```python
from build123d import *

# Parameters (mm, degrees)
SKETCH1_R           = 6.8961
SKETCH1_R_2         = 2.3241
BOSS_EXTRUDE1_DEPTH = 2.794
SKETCH2_R           = 2.3241
BOSS_EXTRUDE2_DEPTH = 0.762
BOSS_EXTRUDE3_DEPTH = 1.651
SKETCH5_R           = 8.206879239
SKETCH5_R_2         = 3.9875
CUT_EXTRUDE1_DEPTH  = 11.144891642
SKETCH6_R           = 4.9875
SKETCH6_R_2         = 3.9875
BOSS_EXTRUDE4_DEPTH = 1
FILLET1_R           = 0.2
SKETCH7_R           = 3.9875
BOSS_EXTRUDE5_DEPTH = 2.5


with BuildPart() as part:
    # Sketch1 → Boss-Extrude1 (new body)
    with BuildSketch(Plane(origin=(0, 0, 0), x_dir=(1, 0, 0), z_dir=(0, 1, 0))):
        with Locations(Location((0, 0, 0), (0, 0, 270))):
            Circle(SKETCH1_R)
        with Locations(Location((0, 0, 0), (0, 0, 270))):
            Circle(SKETCH1_R_2, mode=Mode.SUBTRACT)
    extrude(amount=BOSS_EXTRUDE1_DEPTH)

    # Sketch2 → Boss-Extrude2 (add)
    with BuildSketch(Plane.XZ):
        with Locations(Location((0, 0, 0), (0, 0, 270))):
            Circle(SKETCH2_R)
    extrude(amount=-BOSS_EXTRUDE2_DEPTH)

    # Sketch3 → Boss-Extrude3 (add)
    with BuildSketch(Plane(origin=(0, 0.762, 0), x_dir=(1, 0, 0), z_dir=(0, 1, 0))):
        with BuildLine():
            Line((-0.495805164, 1.156686678), (0.614449488, 1.120298857))
            ThreePointArc((0.614449488, 1.120298857), (0.708812351, 1.091670316), (0.776218716, 1.01969584))
            Line((0.776218716, 1.01969584), (1.299833265, 0.039993196))
            ThreePointArc((1.299833265, 0.039993196), (1.322221652, -0.056041711), (1.293593111, -0.150404573))
            Line((1.293593111, -0.150404573), (0.706953007, -1.093719397))
            ThreePointArc((0.706953007, -1.093719397), (0.634978532, -1.161125762), (0.538943625, -1.183514149))
            Line((0.538943625, -1.183514149), (-0.571311028, -1.147126328))
            ThreePointArc((-0.571311028, -1.147126328), (-0.66567389, -1.118497787), (-0.733080255, -1.046523312))
            Line((-0.733080255, -1.046523312), (-1.256694804, -0.066820667))
            ThreePointArc((-1.256694804, -0.066820667), (-1.279083191, 0.02921424), (-1.25045465, 0.123577102))
            Line((-1.25045465, 0.123577102), (-0.663814546, 1.066891925))
            ThreePointArc((-0.663814546, 1.066891925), (-0.591840071, 1.134298291), (-0.495805164, 1.156686678))
        make_face()
    extrude(amount=BOSS_EXTRUDE3_DEPTH)

    # Sketch5 → Cut-Extrude1 (cut, through all)
    with BuildSketch(Plane(origin=(0, 2.794, 0), x_dir=(1, 0, 0), z_dir=(0, 1, 0))):
        Circle(SKETCH5_R)
        with Locations(Location((0, 0, 0), (0, 0, 270))):
            Circle(SKETCH5_R_2, mode=Mode.SUBTRACT)
    extrude(amount=-CUT_EXTRUDE1_DEPTH, mode=Mode.SUBTRACT)

    # Sketch6 → Boss-Extrude4 (add)
    with BuildSketch(Plane(origin=(0, 2.794, 0), x_dir=(1, 0, 0), z_dir=(0, 1, 0))):
        with Locations(Location((0, 0, 0), (0, 0, 270))):
            Circle(SKETCH6_R)
        with Locations(Location((0, 0, 0), (0, 0, 270))):
            Circle(SKETCH6_R_2, mode=Mode.SUBTRACT)
    extrude(amount=-BOSS_EXTRUDE4_DEPTH)

    # Fillet1
    fillet1_edges = [part.edges().sort_by_distance(p)[0] for p in [
        (0.708812351, 2.413, -1.091670316),
        (0.059322162, 2.413, -1.138492768),
        (-0.591840071, 2.413, -1.134298291),
        (-0.957134598, 2.413, -0.595234514),
        (-1.279083191, 2.413, -0.02921424),
        (-0.99488753, 2.413, 0.556671989),
        (-0.66567389, 2.413, 1.118497787),
        (-0.016183701, 2.413, 1.165320239),
        (0.634978532, 2.413, 1.161125762),
        (1.000273059, 2.413, 0.622061985),
        (1.322221652, 2.413, 0.056041711),
        (1.038025991, 2.413, -0.529844518),
    ]]
    fillet(fillet1_edges, radius=FILLET1_R)

    # Sketch7 → Boss-Extrude5 (add)
    with BuildSketch(Plane.XZ):
        with Locations(Location((0, 0, 0), (0, 0, 90))):
            Circle(SKETCH7_R)
    extrude(amount=BOSS_EXTRUDE5_DEPTH)


solid = part.part
```
The listing builds one solid part. Answer for the finished solid, in the listing's coordinates (mm). A direction names the side the tool comes from. Coordinates: 2 decimals unless noted, no trailing zeros. Write each loop counter-clockwise with the first axis right and the second up, starting at its lowest first coordinate (ties: lowest second). Pieces come first, ordered by that corner, then holes. Notation, with made-up numbers: (-10.75, -2.5) - (-4.75, -2.5) arc R23 cw to (-4.75, 25.5) - close; hole circle Ø7 at (7.25, 23). An arc over 180 degrees is marked (long way). Return JSON: item names as keys, results as strings. Group by question number.
Q1. The part is cut by section A-A on y = 1.65. State how many separate pieces and enclosed holes the cut face has, and give its area (3 significant figures).
Q2. Which of the six approach directions +Z, -Z, +X, -X, +Y, -Y give full straight-line access (tool end or side, diameter ignored) to faces 1 (the flat face through (0, 2.413, 0)), 2 (the flat face through (-1, 2.794, -2.3))?
Q3. The part is cut by section D-D on y = -0.35. Write down the section's boundary in (x, z) (1 decimal).
Q4. Find the intervals of material crossed by line 1 along X through (y, z) = (2.3, 0); line 2 along Y through (x, z) = (4.25, -1); line 3 along Y through (x, z) = (-0.25, 0.5), in increasing order. Write a range as [from, to].
Q5. Flat-ended cylindrical pins translate along their axes: pin 1 Ø2.5 at (x, z) = (-0.5, 0) entering from +Y; pin 2 Ø1.5 at (x, y) = (-3.5, -0.5) entering from -Z. Find the tip coordinate at first contact, or state that the pin passes through.
Q6. The part is cut by section C-C on z = 1.75. Write down the section's boundary in (x, y), and give its area (3 significant figures).
Q7. For a pull along X with two mould halves and no side action, classify faces 3 (the flat face through (-0.991, 1.477, 0.564)), 4 (the cylindrical face through (1.498, 2.301, 4.757)), 5 (the flat face through (-4, 1.794, -2)) as +X half, -X half, draft (parallel to the pull), parting line (faces both ways), or undercut.
Q8. The part is cut by section B-B on x = 1.5. Write down the section's boundary in (y, z), and give its area (3 significant figures).
Evaluation:
{
 "1": {"separate pieces": "2", "enclosed holes": "1", "area": "37.6 mm2"},
 "2": {"face 1": "+Y", "face 2": "+Z, -Z, +X, -X, +Y"},
 "3": {"outline": "circle Ø8 at (0, 0)"},
 "4": {"line 1": "x = [-4.99, -2.32], [-1.26, 1.29], [2.32, 4.99]", "line 2": "y = [1.79, 2.79]", "line 3": "y = [-2.5, 2.41]"},
 "5": {"pin 1": "stops at y = 2.41", "pin 2": "stops at z = -2.89"},
 "6": {"outline": "(-4.67, 1.79) - (-3.58, 1.79) - (-3.58, -2.5) - (3.58, -2.5) - (3.58, 1.79) - (4.67, 1.79) - (4.67, 2.79) - (1.53, 2.79) - (1.53, 0.76) - (-1.53, 0.76) - (-1.53, 2.79) - (-4.67, 2.79) - close", "area": "33.9 mm2"},
 "7": {"face 3": "undercut", "face 4": "parting line", "face 5": "draft"},
 "8": {"outline": "(-2.5, -3.69) - (1.79, -3.69) - (1.79, -4.76) - (2.79, -4.76) - (2.79, -1.78) - (0.76, -1.78) - (0.76, 1.78) - (2.79, 1.78) - (2.79, 4.76) - (1.79, 4.76) - (1.79, 3.69) - (-2.5, 3.69) - close", "area": "34.0 mm2"}
}
